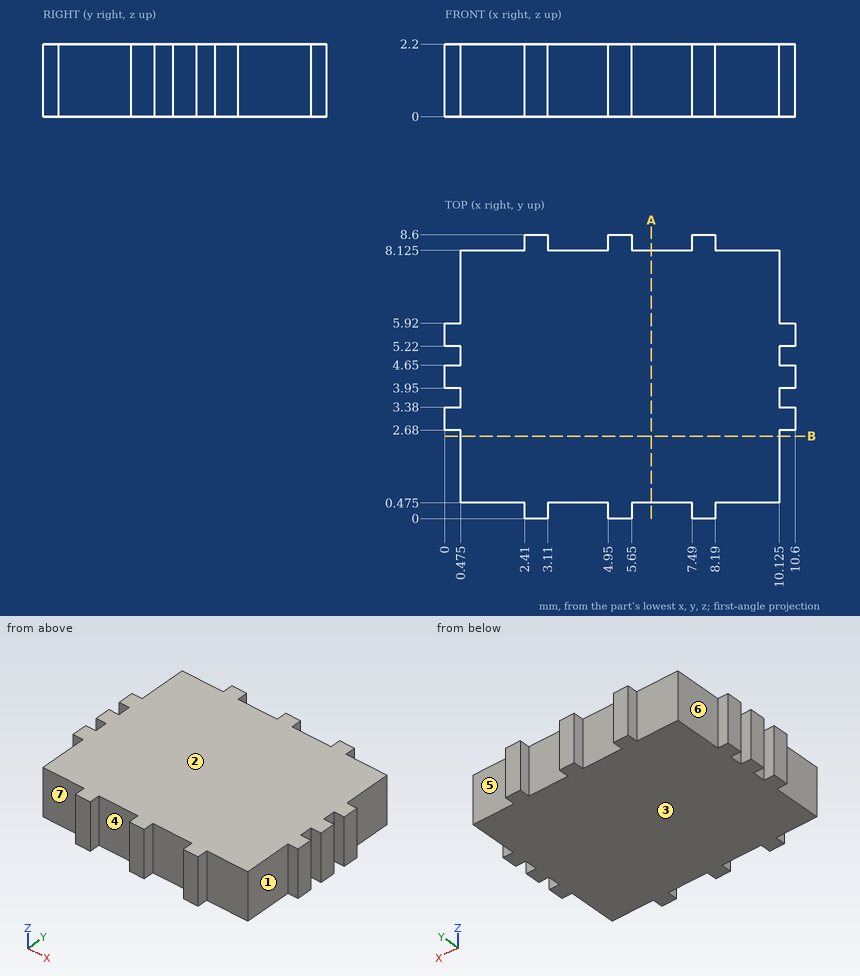
Here's the drawing with two shaded views (mm, measured from the low corner). I have some questions. A direction names the side the tool comes from. Round coordinates to 2 decimals unless told otherwise and drop trailing zeros. Loops run counter-clockwise (first coordinate to the right, second up) from the corner with the lowest first, then second, coordinate; pieces in that order, holes last. Notation, with made-up numbers: M 43.25,71 L 65.25,71 A23 cw 65.25,92 Z; hole C 68,16.5 d3. An arc over 180 degrees is marked long. Answer as a JSON object with one key per item and string values. Group by question number.
Q1. On a 3-axis mill with a long thin cutter (end or side, diameter ignored), from which of +Z, -Z, +X, -X, +Y, -Y can I reach the whole of each face in a straight line? I mean the marked faces 4, 5, 6 and 7. Say none if no direction works.
Q2. Please list where these lines run through material, in increasing order: L1, parallel to Y at x = 10.25, z = 0.95; L2, parallel to Y at x = 6, z = 1.3 (3 decimals); L3, parallel to X at y = 1.5, z = 0.8 (3 decimals).
Q3. Will these pins go through, and if not, where does the flat tip stop? pin 1 (0.5 mm diameter, centred on y = 0, z = 1, fed in from -X); pin 2 (0.9 mm diameter, centred on x = 4, z = 1, fed in from +Y) (3 decimals); pin 3 (0.5 mm diameter, centred on y = 3.5, z = 1.5, fed in from -X); pin 4 (0.7 mm diameter, centred on y = 7.5, z = 1.5, fed in from -X) (3 decimals).
Q4. Imagine slicing it at A-A, the plane x = 6.25. Please give me the cut outline in (y, z) (3 decimals).
Q5. Imagine slicing it at B-B, the plane y = 2.5. Please give me the cut outline in (x, z) (3 decimals), then the cut area to 3 significant figures.
Q6. We'd pull the mould along Z, two halves only. Please class the marked faces 1, 2 and 3: +Z half, -Z half, draft (parallel to the pull), parting line (faces both ways), or undercut.
Findings:
{
 "1": {"face 4": "+Z, -Z, -Y", "face 5": "+Z, -Z, +X, +Y", "face 6": "+Z, -Z, -X, +Y", "face 7": "+Z, -Z, -X, -Y"},
 "2": {"L1": "y = 2.68 to 3.38, 3.95 to 4.65, 5.22 to 5.92", "L2": "y = 0.475 to 8.125", "L3": "x = 0.475 to 10.125"},
 "3": {"pin 1": "stops at x = 2.41", "pin 2": "stops at y = 8.125", "pin 3": "stops at x = 0", "pin 4": "stops at x = 0.475"},
 "4": {"outline": "M 0.475,0 L 8.125,0 L 8.125,2.2 L 0.475,2.2 Z"},
 "5": {"outline": "M 0.475,0 L 10.125,0 L 10.125,2.2 L 0.475,2.2 Z", "area": "21.2 mm2"},
 "6": {"face 1": "draft", "face 2": "+Z half", "face 3": "-Z half"}
}
